```python
from build123d import *

# Parameters (mm, degrees)
SKETCH2_W           = 100.33
SKETCH2_H           = 25.4
BOSS_EXTRUDE1_DEPTH = 3.175
SKETCH3_R           = 3.81
CUT_EXTRUDE1_DEPTH  = 4.175


with BuildPart() as part:
    # Sketch2 → Boss-Extrude1 (new body)
    with BuildSketch(Plane(origin=(0, 0, 0), x_dir=(1, 0, 0), z_dir=(0, 1, 0))):
        Rectangle(SKETCH2_W, SKETCH2_H)
    extrude(amount=BOSS_EXTRUDE1_DEPTH)

    # Sketch3 → Cut-Extrude1 (cut, through all)
    with BuildSketch(Plane(origin=(0, 3.175, 0), x_dir=(1, 0, 0), z_dir=(0, 1, 0))):
        with Locations((-43.434, -7.62)):
            Circle(SKETCH3_R)
        with Locations((-33.274, -7.62)):
            Circle(SKETCH3_R)
        with Locations((-23.114, -7.62)):
            Circle(SKETCH3_R)
        with Locations((-12.954, -7.62)):
            Circle(SKETCH3_R)
        with Locations((-2.794, -7.62)):
            Circle(SKETCH3_R)
        with Locations((7.366, -7.62)):
            Circle(SKETCH3_R)
        with Locations((17.526, -7.62)):
            Circle(SKETCH3_R)
        with Locations((27.686, -7.62)):
            Circle(SKETCH3_R)
        with Locations((37.846, -7.62)):
            Circle(SKETCH3_R)
    extrude(amount=-CUT_EXTRUDE1_DEPTH, mode=Mode.SUBTRACT)


solid = part.part
```
Can you work these out from the model? Positions are in its coordinate system, mm. Coordinates: 2 decimals unless noted, no trailing zeros. Loops run counter-clockwise (first coordinate to the right, second up) from the corner with the lowest first, then second, coordinate; pieces in that order, holes last. Notation, with made-up numbers: (4, 72.25) - (61, 72.25) arc R19 cw to (61, 95.25) - close; hole circle Ø5 at (-38.75, 82). An arc over 180 degrees is marked (long way). Use a Markdown table: item, result.
Item 1: Will this pin go through, and if not, where does the flat tip stop? pin 1 (10 mm diameter, centred on x = 37.846, z = 7.62, fed in from -Y).
Numbers:
| item | result |
|---|---|
| pin 1 | stops at y = 0 |
Item 2: I want a section at A-A on x = -15. Please give me the cut outline in (y, z) (3 decimals).
Numbers:
| item | result |
|---|---|
| outline | (0, -12.7) - (3.175, -12.7) - (3.175, 4.406) - (0, 4.406) - close; (0, 10.834) - (3.175, 10.834) - (3.175, 12.7) - (0, 12.7) - close |
Item 3: I want a section at B-B on y = 0.7. Give the number of separate pieces and of enclosed holes in the cut face, and give its area (3 significant figures).
Numbers:
| item | result |
|---|---|
| separate pieces | 1 |
| enclosed holes | 9 |
| area | 2,140 mm2 |
Item 4: I want a section at D-D on x = -44. Please give me the cut outline in (y, z) (3 decimals), and give its area (3 significant figures).
Numbers:
| item | result |
|---|---|
| outline | (0, -12.7) - (3.175, -12.7) - (3.175, 3.852) - (0, 3.852) - close; (0, 11.388) - (3.175, 11.388) - (3.175, 12.7) - (0, 12.7) - close |
| area | 56.7 mm2 |
Item 5: If I drill on probe 1 along Z at (x, y) = (27.5, 0.9); probe 2 along Z at (x, y) = (25.5, 2.7), over which ranges is the centre line in solid material (lowest first)? Write a range as from..to.
Numbers:
| item | result |
|---|---|
| probe 1 | z = -12.7..3.81, 11.43..12.7 |
| probe 2 | z = -12.7..4.5, 10.74..12.7 |
Item 6: We'd pull the mould along X, two halves only. Please class faces 1 (the face through (50.165, 2, 0)), 2 (the face through (-1, 2, -12.7)), 3 (the face through (-47.24, 1.61, 7.45)): released by +X, released by -X, zero draft, split by the parting line, or undercut.
Numbers:
| item | result |
|---|---|
| face 1 | released by +X |
| face 2 | zero draft |
| face 3 | undercut |
